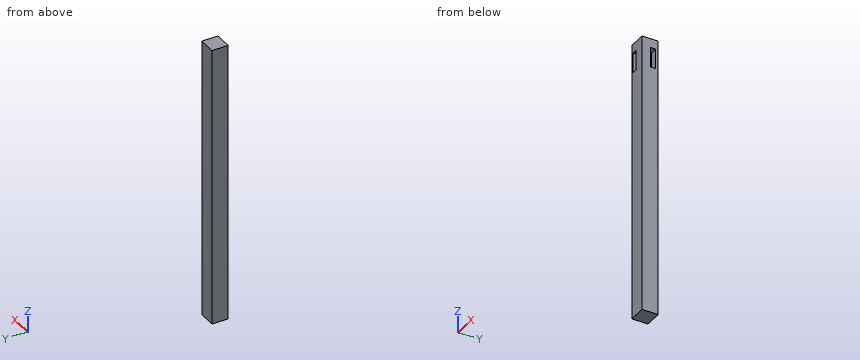
```python
from build123d import *

# Parameters (mm, degrees)
F0_W     = 44.45
F0_H     = 41.148
F1_DEPTH = 355.6
F2_W     = 12.7
F2_H     = 50.8
F3_DEPTH = 19.05
F4_W     = 12.7
F4_H     = 50.8
F5_DEPTH = 19.05


with BuildPart() as f1:
    # F0 (on Top) → F1 (new body, symmetric)
    with BuildSketch(Plane.XY):
        with Locations((-5.032887, 11.366384)):
            Rectangle(F0_W, F0_H)
    extrude(amount=F1_DEPTH, both=True)

    # F2 (on face) → F3 (cut)
    with BuildSketch(Plane.XZ.offset(9.207616)):
        with Locations((-14.557887, 307.34)):
            Rectangle(F2_W, F2_H)
    extrude(amount=-F3_DEPTH, mode=Mode.SUBTRACT)

    # F4 (on face) → F5 (cut)
    with BuildSketch(Plane.YZ.offset(17.192113)):
        with Locations((19.240384, 307.34)):
            Rectangle(F4_W, F4_H)
    extrude(amount=-F5_DEPTH, mode=Mode.SUBTRACT)


with BuildPart() as f6_1:
    # F6: copy of F1
    add(f1.part)


with BuildPart() as f8_1:
    # F8: copy of F1
    add(f1.part)


with BuildPart() as f10_1:
    # F10: copy of F1
    add(f1.part)


solid = f1.part
```
Source: CAD feature listing. Evaluate the final solid. Frame: model axes, mm. Give positions to 0.01 mm unless a question says otherwise; leave off trailing zeros. Loops run counter-clockwise (first coordinate to the right, second up) from the corner with the lowest first, then second, coordinate; pieces in that order, holes last. Notation, with made-up numbers: (-1.75, 30) -> (49.25, 30) arc R20 ccw to (49.25, 50) -> close; hole circle Ø11 at (-15, -7.5). An arc over 180 degrees is marked (long way). Use a Markdown table: item, result. Add a question column.
(1) Section query A-A (x = 10.5). Output: boundary loops of the cut face in (y, z), then the cut area to 3 significant figures.
(2) First-contact query: pin 1 Ø6.5 at (x, z) = (-16, 300.5) entering from -Y; pin 2 Ø10 at (y, z) = (20.5, 307) entering from +X. Flat tips, straight axial feed; report the tip coordinate or a pass-through.
(3) Ray query, line 1 (Z direction, x = 8.5, y = 13); line 2 (Y direction, x = 14.5, z = 306). Return the intervals inside material, ascending.
Checked values:
| question | item | result |
|---|---|---|
| 1 | outline | (-9.21, -355.6) -> (31.94, -355.6) -> (31.94, 355.6) -> (-9.21, 355.6) -> close; hole (12.89, 281.94) -> (25.59, 281.94) -> (25.59, 332.74) -> (12.89, 332.74) -> close |
| 1 | area | 28,600 mm^2 |
| 2 | pin 1 | y = 9.84 |
| 2 | pin 2 | x = -1.86 |
| 3 | line 1 | -355.6 to 281.94, 332.74 to 355.6 |
| 3 | line 2 | -9.21 to 12.89, 25.59 to 31.94 |
